Here's how the part is built. I have some questions about the finished solid (model axes, mm). A direction names the side the tool comes from. Give positions to 0.01 mm unless a question says otherwise; leave off trailing zeros. Write each loop counter-clockwise with the first axis right and the second up, starting at its lowest first coordinate (ties: lowest second). Pieces come first, ordered by that corner, then holes. Notation, with made-up numbers: (31, -37) - (81, -37) arc R13 ccw to (81, -25) - close; hole circle Ø7 at (1, 52). An arc over 180 degrees is marked (long way). Use a Markdown table: item, result.
Autodesk Inventor part; units mm, degrees
ref_plane "YZ Plane" through (0, 0, 0) normal (1, 0, 0) x (0, 1, 0)
ref_plane "XZ Plane" through (0, 0, 0) normal (0, 1, 0) x (-1, 0, 0)
ref_plane "XY Plane" through (0, 0, 0) normal (0, 0, 1) x (1, 0, 0)
sketch "草图1" plane through (0, 0, 0) normal (0, 1, 0) x (-1, 0, 0)
  line L0 (55.7629, 0) -> (-64.7988, 0)
  line L1 (26.8095, -22.5) -> (-26.8095, -22.5)
  line L2 (26.8095, 22.5) -> (-29.1705, 22.5)
  line L3 (0, -45.1984) -> (0, 63.6584)
  arc A0 (30, 7) -> (30, -7) centre (30, 0) ccw
  arc A1 (-30, -7) -> (-30, 7) centre (-30, 0) ccw
  line L4 (30, -7) -> (34.2929, -7)
  line L5 (30, 7) -> (34.2929, 7)
  line L6 (-30, -7) -> (-34.2929, -7)
  line L7 (-30, 7) -> (-34.2929, 7)
  arc A2 (26.8095, -22.5) -> (34.2929, -7) centre (0, 0) ccw
  arc A3 (34.2929, 7) -> (26.8095, 22.5) centre (0, 0) ccw
  arc A4 (-26.8095, 22.5) -> (-34.2929, 7) centre (0, 0) ccw
  arc A5 (-34.2929, -7) -> (-26.8095, -22.5) centre (0, 0) ccw
  dimension "d1" = 45
  dimension "d2" = 14
  dimension "d3" = 60
extrude "拉伸1" add sketch "草图1" along normal blind 6
sketch "草图2" plane through (0, 6, 0) normal (0, 1, 0) x (1, 0, 0)
  arc A0 (34.2929, 7) -> (26.8095, 22.5) centre (0, 0) ccw
  circle A1 centre (0, 0) radius 17.5
  dimension "d6" = 35
extrude "拉伸2" add sketch "草图2" along normal blind 40
sketch "草图3" plane through (0, 0, 0) normal (0, -1, 0) x (1, 0, 0)
  arc A0 (-34.2929, -7) -> (-26.8095, -22.5) centre (0, 0) ccw
  circle A1 centre (0, 0) radius 6
  dimension "d9" = 12
extrude "拉伸3" cut sketch "草图3" against normal blind 60
sketch "草图4" plane through (0, 6, 0) normal (0, 1, 0) x (1, 0, 0)
  circle A0 centre (0, 0) radius 17.5
  arc A1 (-26.8095, 22.5) -> (-34.2929, 7) centre (0, 0) ccw
  line L0 (-34.2929, 7) -> (-30, 7)
  arc A2 (-30, -7) -> (-30, 7) centre (-30, 0) ccw
  line L1 (-30, -7) -> (-34.2929, -7)
  arc A3 (-34.2929, -7) -> (-26.8095, -22.5) centre (0, 0) ccw
  arc A4 (26.8095, -22.5) -> (34.2929, -7) centre (0, 0) ccw
  line L2 (34.2929, -7) -> (30, -7)
  arc A5 (30, 7) -> (30, -7) centre (30, 0) ccw
  line L3 (30, 7) -> (34.2929, 7)
  arc A6 (34.2929, 7) -> (26.8095, 22.5) centre (0, 0) ccw
  line L4 (-33.2265, 11) -> (-13.6107, 11)
  line L5 (13.6107, 11) -> (33.2265, 11)
  line L6 (-33.2265, -11) -> (-13.6107, -11)
  line L7 (13.6107, -11) -> (33.2265, -11)
  line L8 (-37.479, 0) -> (55.827, 0)
  line L9 (0, 23.5503) -> (0, -22.0958)
  dimension "d12" = 22
extrude "拉伸4" add sketch "草图4" along normal blind 8 contours L8 A5 L2 A4 L7 A0 | A0 L5 A6 L3 A5 L8 | L8 A2 L0 A1 L4 A0 | A0 L6 A3 L1 A2 L8
sketch "草图5" plane through (0, 46, 0) normal (0, 1, 0) x (1, 0, 0)
  circle A0 centre (0, 0) radius 6
  circle A1 centre (0, 0) radius 17.5
  circle A2 centre (0, 0) radius 13
  dimension "d15" = 26
extrude "拉伸5" cut sketch "草图5" against normal blind 26 contours A2
sketch "草图6" plane through (0, 0, 0) normal (0, 0, 1) x (1, 0, 0)
  point P0 (0, 0)
sketch "草图7" plane through (0, 0, 0) normal (0, 0, 1) x (1, 0, 0)
  line L0 (0, 0) -> (0, 58.8844)
  line L1 (-23, 14) -> (-17.5, 14)
  line L2 (-17.5, 14) -> (-17.5, 46)
  line L3 (-17.5, 46) -> (-13, 46)
  line L4 (-13, 46) -> (-13, 20)
  line L5 (-13, 20) -> (-6, 20)
  line L6 (-6, 20) -> (-6, 0)
  line L7 (-6, 0) -> (-23, 0)
  line L8 (-23, 0) -> (-23, 14)
  line L9 (17.5, 14) -> (23, 14)
  line L10 (23, 14) -> (23, 0)
  line L11 (23, 0) -> (6, 0)
  line L12 (6, 0) -> (6, 20)
  line L13 (6, 20) -> (13, 20)
  line L14 (13, 20) -> (13, 46)
  line L15 (13, 46) -> (17.5, 46)
  line L16 (17.5, 46) -> (17.5, 14)
  circle A0 centre (0, 34) radius 8
  line L17 (-13, 46) -> (13, 46)
  dimension "d18" = 16
  dimension "d19" = 12
extrude "拉伸6" cut sketch "草图7" against normal blind 26 contours A0 L0 | L0 A0
sketch "草图8" plane through (0, 0, 0) normal (0, 0, 1) x (1, 0, 0)
  line L0 (-23, 14) -> (-17.5, 14)
  line L1 (-17.5, 14) -> (-17.5, 46)
  line L2 (-17.5, 46) -> (-13, 46)
  line L3 (-13, 46) -> (-13, 20)
  line L4 (-13, 20) -> (-6, 20)
  line L5 (-6, 20) -> (-6, 0)
  line L6 (-6, 0) -> (-23, 0)
  line L7 (-23, 0) -> (-23, 14)
  line L8 (17.5, 14) -> (23, 14)
  line L9 (23, 14) -> (23, 0)
  line L10 (23, 0) -> (6, 0)
  line L11 (6, 0) -> (6, 20)
  line L12 (6, 20) -> (13, 20)
  line L13 (13, 20) -> (13, 46)
  line L14 (13, 46) -> (17.5, 46)
  line L15 (17.5, 46) -> (17.5, 14)
  line L16 (-23, 14) -> (-17.5, 14)
  line L17 (-17.5, 14) -> (-17.5, 46)
  line L18 (-17.5, 46) -> (-13, 46)
  line L19 (-13, 46) -> (-13, 20)
  line L20 (-13, 20) -> (-6, 20)
  line L21 (-6, 20) -> (-6, 0)
  line L22 (-6, 0) -> (-23, 0)
  line L23 (-23, 0) -> (-23, 14)
  line L24 (17.5, 14) -> (23, 14)
  line L25 (23, 14) -> (23, 0)
  line L26 (23, 0) -> (6, 0)
  line L27 (6, 0) -> (6, 20)
  line L28 (6, 20) -> (13, 20)
  line L29 (13, 20) -> (13, 46)
  line L30 (13, 46) -> (17.5, 46)
  line L31 (17.5, 46) -> (17.5, 14)
  line L32 (-23, 14) -> (-17.5, 14)
  line L33 (-17.5, 14) -> (-17.5, 46)
  line L34 (-17.5, 46) -> (-13, 46)
  line L35 (-13, 46) -> (-13, 20)
  line L36 (-13, 20) -> (-6, 20)
  line L37 (-6, 20) -> (-6, 0)
  line L38 (-6, 0) -> (-23, 0)
  line L39 (-23, 0) -> (-23, 14)
  line L40 (17.5, 14) -> (23, 14)
  line L41 (23, 14) -> (23, 0)
  line L42 (23, 0) -> (6, 0)
  line L43 (6, 0) -> (6, 20)
  line L44 (6, 20) -> (13, 20)
  line L45 (13, 20) -> (13, 46)
  line L46 (13, 46) -> (17.5, 46)
  line L47 (17.5, 46) -> (17.5, 14)
  line L48 (0, 49.6225) -> (0, -12.8831)
  line L49 (-8, 46) -> (8, 46)
  line L50 (8, 46) -> (8, 20)
  line L51 (8, 20) -> (-8, 20)
  line L52 (-8, 20) -> (-8, 46)
  point P0 (0, 0)
  dimension "d22" = 16
  dimension "d23" = 26
extrude "拉伸7" cut sketch "草图8" along normal blind 26 contours L4 L52 L49 L48 L51 | L48 L49 L50 L12 L51
Item 1: For faces 5 (the flat face through (32, 7, -7)), 6 (the flat face through (-24, 10, -11)), 7 (the flat face through (-3.1, 20, 5.4)), 8 (the flat face through (0, 6, -18)), which set-ups out of +Z, -Z, +X, -X, +Y, -Y let a thin tool reach every point of the face, with its end or its side?
Values:
| item | result |
|---|---|
| face 5 | +X, +Y, -Y |
| face 6 | -Z, -X, +Y |
| face 7 | +Y |
| face 8 | -Z, +Y |
Item 2: I need wall thicknesses on line 1 along X through (y, z) = (35, 0); line 2 along Z through (x, y) = (0, 7.75); line 3 along X through (y, z) = (9, 0). Which ranges of each line are inside material? Lowest first, please. Write a range as [from, to].
Values:
| item | result |
|---|---|
| line 1 | x = [-17.5, -13], [13, 17.5] |
| line 2 | z = [-17.5, -6], [6, 17.5] |
| line 3 | x = [-23, -6], [6, 23] |
Item 3: If we section it at C-C, the plane x = 9: Write out the boundary of the cut face in (y, z).
Values:
| item | result |
|---|---|
| outline | (0, -22.5) - (6, -22.5) - (6, -15.01) - (46, -15.01) - (46, -9.38) - (20, -9.38) - (20, 9.38) - (46, 9.38) - (46, 15.01) - (6, 15.01) - (6, 22.5) - (0, 22.5) - close |
Item 4: If we section it at D-D, the plane y = 23: Write out the boundary of the cut face in (x, z), plus the area to 3 significant figures.
Values:
| item | result |
|---|---|
| outline | (-8, 10.25) - (-8, 15.56) arc R17.5 ccw (long way) to (8, 15.56) - (8, 10.25) arc R13 cw (long way) to start |
| area | 355 mm2 |
Item 5: If we section it at B-B, the plane y = 34: Write out the boundary of the cut face in (x, z).
Values:
| item | result |
|---|---|
| outline | (-8, -15.56) - (-8, -10.25) arc R13 cw to (-8, 10.25) - (-8, 15.56) arc R17.5 ccw to start; (8, -15.56) arc R17.5 ccw to (8, 15.56) - (8, 10.25) arc R13 cw to (8, -10.25) - close |
Item 6: Thinking about a two-plate mould opening in Z: for faces 1 (the cylindrical face through (32.264, 3.791, -13.567)), 2 (the flat face through (-32, 7, -7)), 3 (the flat face through (8, 33, 13)), 4 (the cylindrical face through (-32.264, 3.791, 13.567)), which applies, +Z half, -Z half, draft (parallel to the pull), parting line (faces both ways), or undercut?
Values:
| item | result |
|---|---|
| face 1 | -Z half |
| face 2 | undercut |
| face 3 | draft |
| face 4 | +Z half |
Item 7: If we section it at A-A, the plane x = 0: Write out the boundary of the cut face in (y, z).
Values:
| item | result |
|---|---|
| outline | (0, -22.5) - (6, -22.5) - (6, -17.5) - (26, -17.5) - (26, -13) - (20, -13) - (20, -6) - (0, -6) - close; (0, 6) - (20, 6) - (20, 17.5) - (6, 17.5) - (6, 22.5) - (0, 22.5) - close; (42, -17.5) - (46, -17.5) - (46, -13) - (42, -13) - close |
Item 8: Will these pins go through, and if not, where does the flat tip stop? pin 1 Ø4.5 at (y, z) = (35, 13.5) entering from -X; pin 2 Ø1.3 at (x, y) = (32, 7) entering from -Z; pin 3 Ø9 at (x, y) = (-19, 11.5) entering from +Z; pin 4 Ø8 at (x, y) = (1, 33.5) entering from +Z.
Values:
| item | result |
|---|---|
| pin 1 | stops at x = -13.4 |
| pin 2 | stops at z = -11 |
| pin 3 | stops at z = 11 |
| pin 4 | passes through |
